For this review, take the finished solid that the model builds, in its own axes (mm). Coordinates: 2 decimals unless noted, no trailing zeros. Order: outer loops, then holes, each group sorted by start corner. A loop starts at its lowest first (then second) coordinate and runs counter-clockwise, first axis right, second up. Notation, with made-up numbers: (88, -30.5) - (133, -30.5) arc R22 ccw to (133, -3.5) - close; hole circle Ø4 at (-2, 6.5). An arc over 180 degrees is marked (long way). One line per item, written item: value. Start each with the question number.
(1) Consider section B-B on x = 413. Write out the cut boundary in (y, z).
(2) Clearance check with flat-ended pins moving along their axes: pin 1 (20 mm diameter, centred on x = -487, z = -189.5, fed in from +Y); pin 2 (4 mm diameter, centred on x = -281, y = 6, fed in from -Z); pin 3 (12 mm diameter, centred on x = 488.5, z = -113.5, fed in from -Y). State where each tip first meets the part, or that it passes through.
(3) Consider section A-A on z = -328. Write out the cut boundary in (x, y).
(4) To check wall thickness, follow line 1 along X through (y, z) = (34, -319); line 2 along Z through (x, y) = (288, 63.5); line 3 along Y through (x, z) = (-297.5, 2.5). State the ranges of each line that lie inside material, in increasing order.
(5) Consider section C-C on y = -19. Write out the cut boundary in (x, z), then the cut area to 3 significant figures.
```python
from build123d import *

# Parameters (mm, degrees)
F1_DEPTH = 500
F2_W     = 40
F2_H     = 60
F3_DEPTH = 400


# Not quite as in the source:
# - a pattern or mirror of a feature is missing from the dataset's text; its kind, count and spacing are read off the source's solid


with BuildPart() as f1:
    # F0 (on Right) → F1 (new body, symmetric)
    with BuildSketch(Plane.YZ):
        with BuildLine():
            Line((-65, 0), (-5, 0))
            ThreePointArc((-5, 0), (-1.4644660941, 1.4644660941), (0, 5))
            Line((0, 5), (0, 35))
            ThreePointArc((0, 35), (-1.4644660941, 38.5355339059), (-5, 40))
            Line((-5, 40), (-65, 40))
            ThreePointArc((-65, 40), (-68.5355339059, 38.5355339059), (-70, 35))
            Line((-70, 35), (-70, 5))
            ThreePointArc((-70, 5), (-68.5355339059, 1.4644660941), (-65, 0))
        make_face()
    extrude(amount=F1_DEPTH, both=True)

    # F2 (on face) → F3 (join)
    with BuildSketch(Plane(origin=(0, 0, 0), x_dir=(1, 0, 0), z_dir=(0, 0, -1))):
        with Locations((480, 35)):
            Rectangle(F2_W, F2_H)
    f3 = extrude(amount=F3_DEPTH)

    # F3_copies: F3 across plane
    add(f3.mirror(Plane(origin=(0, 0, 0), x_dir=(0, 0, -1), z_dir=(-1, 0, 0))))

    # F4: F1 across plane


with BuildPart() as f1_1:
    add(f1.part)
    add(f1.part.mirror(Plane.XZ))


solid = f1_1.part
```
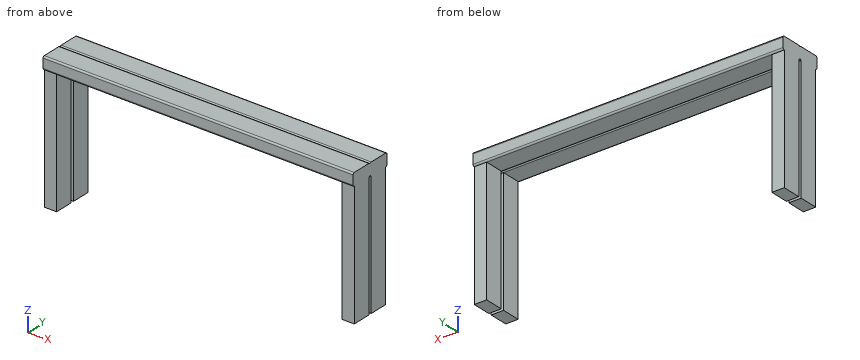
Geometry check:
1. outline: (-70, 5) arc R5 ccw to (-65, 0) - (-5, 0) arc R5 ccw to (0, 5) arc R5 ccw to (5, 0) - (65, 0) arc R5 ccw to (70, 5) - (70, 35) arc R5 ccw to (65, 40) - (5, 40) arc R5 ccw to (0, 35) arc R5 ccw to (-5, 40) - (-65, 40) arc R5 ccw to (-70, 35) - close
2. pin 1: stops at y = 65
2. pin 2: stops at z = 0
2. pin 3: stops at y = -65
3. outline: (-500, -65) - (-460, -65) - (-460, -5) - (-500, -5) - close; (-500, 5) - (-460, 5) - (-460, 65) - (-500, 65) - close; (460, -65) - (500, -65) - (500, -5) - (460, -5) - close; (460, 5) - (500, 5) - (500, 65) - (460, 65) - close
4. line 1: x = -500 to -460, 460 to 500
4. line 2: z = 0 to 40
4. line 3: y = -69.33 to -0.67, 0.67 to 69.33
5. outline: (-500, -400) - (-460, -400) - (-460, 0) - (460, 0) - (460, -400) - (500, -400) - (500, 40) - (-500, 40) - close
5. area: 72,000 mm^2
